from build123d import *

# Parameters (mm, degrees)
CYLINDER001_R     = 1.75
CYLINDER001_DEPTH = 9
CYLINDER_R        = 2.5
CYLINDER_DEPTH    = 3
FILLET_R          = 1


with BuildPart() as cilindro001:
    # Cylinder001 → Cylinder001 (new body)
    with BuildSketch(Plane.XY):
        Circle(CYLINDER001_R)
    extrude(amount=CYLINDER001_DEPTH)


with BuildPart() as fillet_body:
    # Cylinder → Cylinder (new body)
    with BuildSketch(Plane.XY):
        Circle(CYLINDER_R)
    extrude(amount=CYLINDER_DEPTH)

    # Fusion: union Cilindro001
    add(cilindro001.part)

    # Fillet
    fillet_edges = [fillet_body.edges().sort_by_distance(p)[0] for p in [
        (-1.75, 0, 9),
    ]]
    fillet(fillet_edges, radius=FILLET_R)


solid = fillet_body.part
Read the model definition and answer for the solid it produces. Units are mm, in the model's axes. A direction names the side the tool comes from. Coordinates: 2 decimals unless noted, no trailing zeros. Loops run counter-clockwise (first coordinate to the right, second up) from the corner with the lowest first, then second, coordinate; pieces in that order, holes last. Notation, with made-up numbers: (60, 74.5) -> (84, 74.5) arc R10 cw to (84, 87.5) -> close; hole circle Ø3 at (69.25, 66). An arc over 180 degrees is marked (long way). Write item = value, one per line. Start each with the question number.
1) The part is cut by section C-C, the plane y = 1.9. Determine the outline of the cut face in (x, z), plus the area to 3 significant figures.
2) For faces 3 (the face through (-2, -1, 3)), 4 (the face through (0, 0, 9)), determine the directions among +Z, -Z, +X, -X, +Y, -Y from which every point of the face is accessible in a straight line to the end or side of a thin tool.
3) The part is cut by section A-A, the plane x = 2. Determine the outline of the cut face in (y, z), plus the area to 3 significant figures.
4) Given P1, Ø1.5, axis at x = 1.5, z = 8, coming from the -Y side; P2, Ø1, axis at x = -1.5, y = 2, coming from the +Z side, each flat-ended and moving along its own axis, determine where each tip first touches the part or whether it passes through.
5) The mould has two halves that part along Y. Classify faces 1 (the face through (0, 0, 0)), 2 (the face through (1.617, -0.67, 5.465)): pulls with the +Y half, pulls with the -Y half, needs draft (parallel to the pull), parting line crosses it, or undercut.
6) The part is cut by section B-B, the plane z = 5.25. Determine the outline of the cut face in (x, y), plus the area to 3 significant figures.
7) Find the intervals of material crossed by L1, parallel to Z at x = 1.8, y = -0.4; L2, parallel to Y at x = 0, z = 6, in increasing order. Write a range as from..to.
Result:
q1.outline = (-1.62, 0) -> (1.62, 0) -> (1.62, 3) -> (-1.62, 3) -> close
q1.area = 9.75 mm²
q2.face_3 = +Z
q2.face_4 = +Z, +X, -X, +Y, -Y
q3.outline = (-1.5, 0) -> (1.5, 0) -> (1.5, 3) -> (-1.5, 3) -> close
q3.area = 9.00 mm²
q4.P1 = -1.58
q4.P2 = 3
q5.face_1 = needs draft
q5.face_2 = parting line crosses it
q6.outline = circle Ø3.5 at (0, 0)
q6.area = 9.62 mm²
q7.L1 = 0..3
q7.L2 = -1.75..1.75
